For this review, take the finished solid that the model builds, in its own axes (mm). Face numbers are marked on the shaded views. A direction names the side the tool comes from. Round coordinates to 2 decimals unless told otherwise and drop trailing zeros. Order: outer loops, then holes, each group sorted by start corner. A loop starts at its lowest first (then second) coordinate and runs counter-clockwise, first axis right, second up. Notation, with made-up numbers: (3.5, 7) -> (32.5, 7) arc R22 ccw to (32.5, 46) -> close; hole circle Ø2 at (-19, 10). An arc over 180 degrees is marked (long way). Use a Markdown table: item, result. Add a question column.
1) Clearance check with flat-ended pins moving along their axes: P1, Ø15, axis at x = 9, y = -10, coming from the +Z side; P2, Ø1, axis at y = -19, z = 7.5, coming from the -X side; P3, Ø1.1, axis at x = 20.5, y = -1.5, coming from the +Z side; P4, Ø3, axis at x = 21, z = -2, coming from the +Y side. State where each tip first meets the part, or that it passes through.
2) Consider section A-A (x = 36). State the section outline as (y, z) points.
3) Consider section B-B (y = -18.5). State the section outline as (x, z) points.
4) Consider section C-C (z = -1.75). State the section outline as (x, y) points.
5) Machinability: for the marked faces 1, 2, 3 and 4, which of the approach directions +Z, -Z, +X, -X, +Y, -Y give a long, thin tool a straight path to every point of the face, cutting with its end or side? Answer none if there is none.
6) Consider section D-D (x = 7). State the section outline as (y, z) points.
7) Draft analysis for pull direction X (two halves, no side actions). For the marked faces 5, 6 and 7, state which applies: pulls with the +X half, pulls with the -X half, needs draft (parallel to the pull), parting line crosses it, or undercut.
8) Wall thickness on line 1 along Y through (x, z) = (9, 14.95); line 2 along Z through (x, y) = (18, -5); line 3 along Z through (x, y) = (36, -11.5): over which ranges is each line inside the solid? List them lowest first. Write a range as [from, to].
```python
from build123d import *

# Parameters (mm, degrees)
F1_DEPTH = 1.2
F3_DEPTH = 4
F5_DEPTH = 6.5
F7_DEPTH = 13.8
F8_DEPTH = 13.3
F9_DEPTH = 3.5
F10_R    = 1.74999


# Not quite as in the source:
# - a fillet or chamfer is up to 0.001 mm smaller than in the source, because OpenCascade refuses the exact size


with BuildPart() as f1:
    # F0 (on Top) → F1 (new body)
    with BuildSketch(Plane.XY):
        Polygon((9, 0), (0, 0), (0, -20), (45, -20), (45, 0), (36, 0), (22.5, 0), align=None)
    extrude(amount=F1_DEPTH)

    # F2 (on face) → F3 (join)
    with BuildSketch(Plane(origin=(0, 0, 0), x_dir=(1, 0, 0), z_dir=(0, 0, -1))):
        Polygon((22.5, 16.75), (27.5, 16.75), (27.5, 19.25), (17.5, 19.25), (17.5, 16.75), align=None)
    extrude(amount=F3_DEPTH)

    # F4 (on face) → F5 (join)
    with BuildSketch(Plane.XZ.offset(19.25)):
        Polygon((22.5, -3.5), (17.5, -3.5), (17.5, -4), (27.5, -4), (27.5, -3.5), align=None)
    extrude(amount=F5_DEPTH)

    # F6 (on face) → F7 (join)
    with BuildSketch(Plane.XY.offset(1.2)):
        with BuildLine():
            ThreePointArc((44, -10), (36, -2), (28, -10))
            ThreePointArc((28, -10), (36, -18), (44, -10))
        make_face()
        with BuildLine():
            ThreePointArc((42.5, -10), (36, -16.5), (29.5, -10))
            ThreePointArc((29.5, -10), (36, -3.5), (42.5, -10))
        make_face(mode=Mode.SUBTRACT)
        with BuildLine():
            ThreePointArc((17, -10), (14.6568542495, -4.3431457505), (9, -2))
            Line((9, -2), (9, -3.5))
            ThreePointArc((9, -3.5), (13.5961940777, -5.4038059223), (15.5, -10))
            Line((15.5, -10), (17, -10))
        make_face()
        with BuildLine():
            Line((9, -3.5), (9, -2))
            ThreePointArc((9, -2), (3.3431457505, -15.6568542495), (17, -10))
            Line((17, -10), (15.5, -10))
            ThreePointArc((15.5, -10), (4.4038059223, -14.5961940777), (9, -3.5))
        make_face()
    extrude(amount=F7_DEPTH)

    # F8 (add): faces of the model
    f8_faces = [f1.faces().sort_by_distance(p)[0] for p in [
        (9, -10, 1.2),
        (36, -10, 1.2),
    ]]
    extrude(f8_faces, amount=F8_DEPTH)

    # F6 (on face) → F9 (join)
    with BuildSketch(Plane.XY.offset(1.2)):
        Polygon((27.5, -0.25), (22.5, -0.25), (17.5, -0.25), (17.5, -3.75), (27.5, -3.75), align=None)
    extrude(amount=F9_DEPTH)

    # F10 (radius 1.75 in the source; OpenCascade refuses exactly that, so slightly less here)
    f10_edges = [f1.edges().sort_by_distance(p)[0] for p in [
        (27.5, -0.25, 2.95),
        (27.5, -3.75, 2.95),
        (17.5, -0.25, 2.95),
        (17.5, -3.75, 2.95),
    ]]
    fillet(f10_edges, radius=F10_R)


solid = f1.part
```
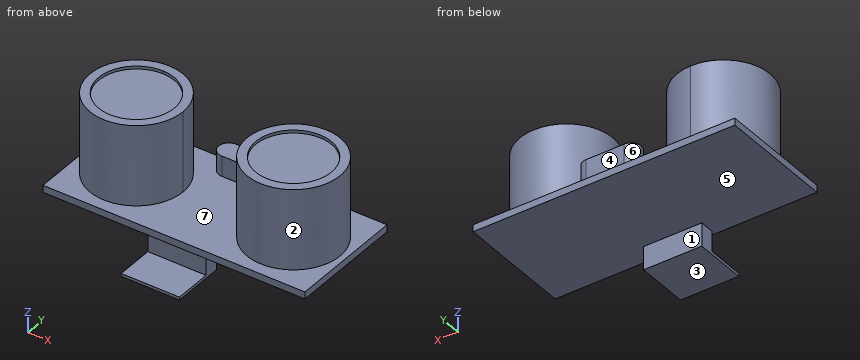
Results list:
| question | item | result |
|---|---|---|
| 1 | P1 | z = 15 |
| 1 | P2 | through |
| 1 | P3 | z = 4.7 |
| 1 | P4 | y = -16.75 |
| 2 | outline | (-20, 0) -> (0, 0) -> (0, 1.2) -> (-2, 1.2) -> (-2, 15) -> (-3.5, 15) -> (-3.5, 14.5) -> (-16.5, 14.5) -> (-16.5, 15) -> (-18, 15) -> (-18, 1.2) -> (-20, 1.2) -> close |
| 3 | outline | (0, 0) -> (17.5, 0) -> (17.5, -4) -> (27.5, -4) -> (27.5, 0) -> (45, 0) -> (45, 1.2) -> (0, 1.2) -> close |
| 4 | outline | (17.5, -19.25) -> (27.5, -19.25) -> (27.5, -16.75) -> (17.5, -16.75) -> close |
| 5 | face 1 | -Z, +X, -X, +Y |
| 5 | face 2 | +Z |
| 5 | face 3 | -Z, +X, -X, +Y, -Y |
| 5 | face 4 | +Z, +X, -X, +Y |
| 6 | outline | (-20, 0) -> (0, 0) -> (0, 1.2) -> (-2.25, 1.2) -> (-2.25, 15) -> (-3.82, 15) -> (-3.82, 14.5) -> (-16.18, 14.5) -> (-16.18, 15) -> (-17.75, 15) -> (-17.75, 1.2) -> (-20, 1.2) -> close |
| 7 | face 5 | needs draft |
| 7 | face 6 | pulls with the -X half |
| 7 | face 7 | undercut |
| 8 | line 1 | [-18, -16.5], [-3.5, -2] |
| 8 | line 2 | [0, 1.2] |
| 8 | line 3 | [0, 14.5] |
